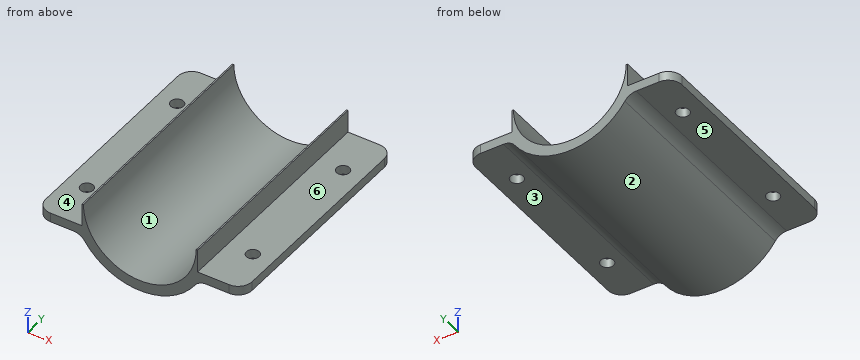
from build123d import *

# Parameters (mm, degrees)
BOSS_EXTRUDE1_DEPTH = 50
SKETCH2_R           = 1.4
CUT_EXTRUDE3_DEPTH  = 2
FILLET2_R           = 3


with BuildPart() as part:
    # Sketch1 → Boss-Extrude1 (new body)
    with BuildSketch(Plane(origin=(0, 0, 0), x_dir=(1, 0, 0), z_dir=(0, 1, 0))):
        with BuildLine():
            Line((-12.6, 0), (-12.6, 5))
            Line((-12.6, 5), (-22.5, 5))
            Line((-22.5, 5), (-22.5, 7))
            Line((-22.5, 7), (-22.1, 7))
            Line((-22.1, 7), (-14.483093592, 7))
            ThreePointArc((-14.483093592, 7), (-13.089113026, 7.343532763), (-12.014384457, 8.295454545))
            ThreePointArc((-12.014384457, 8.295454545), (0, 14.6), (12.014384457, 8.295454545))
            ThreePointArc((12.014384457, 8.295454545), (13.089113026, 7.343532763), (14.483093592, 7))
            Line((14.483093592, 7), (22.1, 7))
            Line((22.1, 7), (22.5, 7))
            Line((22.5, 7), (22.5, 5))
            Line((22.5, 5), (12.6, 5))
            Line((12.6, 5), (12.6, 0))
            Line((12.6, 0), (12.3, 0))
            ThreePointArc((12.3, 0), (0, 12.3), (-12.3, 0))
            Line((-12.3, 0), (-12.6, 0))
        make_face()
    extrude(amount=BOSS_EXTRUDE1_DEPTH)

    # Sketch2 → Cut-Extrude3 (cut)
    with BuildSketch(Plane(origin=(0, 0, -7), x_dir=(-1, 0, 0), z_dir=(0, 0, -1))):
        with Locations((-18.1, 10)):
            Circle(SKETCH2_R)
        with Locations(Location((-18.1, 40, 0), (0, 0, 180))):
            Circle(SKETCH2_R)
        with Locations((18.1, 40)):
            Circle(SKETCH2_R)
        with Locations(Location((18.1, 10, 0), (0, 0, 180))):
            Circle(SKETCH2_R)
    extrude(amount=-CUT_EXTRUDE3_DEPTH, mode=Mode.SUBTRACT)

    # Fillet2
    fillet2_edges = [part.edges().sort_by_distance(p)[0] for p in [
        (-22.5, 0, -6),
        (22.5, 0, -6),
        (22.5, 50, -6),
        (-22.5, 50, -6),
    ]]
    fillet(fillet2_edges, radius=FILLET2_R)


solid = part.part
Could you check a few things on this model? Use its own coordinates, in mm. Face numbers are marked on the shaded views. A direction names the side the tool comes from. Coordinates: 2 decimals unless noted, no trailing zeros. Loops run counter-clockwise (first coordinate to the right, second up) from the corner with the lowest first, then second, coordinate; pieces in that order, holes last. Notation, with made-up numbers: (-19.5, 74.25) -> (22.5, 74.25) arc R9 ccw to (22.5, 90.25) -> close; hole circle Ø6 at (57.5, -31.5). An arc over 180 degrees is marked (long way). Answer in a Markdown table with one row per item.
(1) If I drill on probe 1 along Y at (x, z) = (-18.1, -5.85); probe 2 along X at (y, z) = (41, -9.5); probe 3 along Z at (x, y) = (21, 41.5), over which ranges is the centre line in solid material (lowest first)?
Results found:
| item | result |
|---|---|
| probe 1 | y = 0 to 8.6, 11.4 to 38.6, 41.4 to 50 |
| probe 2 | x = -11.09 to -7.81, 7.81 to 11.09 |
| probe 3 | z = -7 to -5 |
(2) For the marked faces 4, 5 and 6, which set-ups out of +Z, -Z, +X, -X, +Y, -Y let a thin tool reach every point of the face, with its end or its side?
Results found:
| item | result |
|---|---|
| face 4 | +Z, -X, +Y, -Y |
| face 5 | -Z, -X, +Y, -Y |
| face 6 | +Z, +X, +Y, -Y |
(3) Imagine slicing it at C-C (y = 40). List the corners of the cut face in (x, z) for me, plus the area to 3 significant figures.
Results found:
| item | result |
|---|---|
| outline | (-22.5, -7) -> (-19.5, -7) -> (-19.5, -5) -> (-22.5, -5) -> close; (-16.7, -7) -> (-14.48, -7) arc R3 cw to (-12.01, -8.3) arc R14.6 ccw to (12.01, -8.3) arc R3 cw to (14.48, -7) -> (16.7, -7) -> (16.7, -5) -> (12.6, -5) -> (12.6, 0) -> (12.3, 0) arc R12.3 cw to (-12.3, 0) -> (-12.6, 0) -> (-12.6, -5) -> (-16.7, -5) -> close; (19.5, -7) -> (22.5, -7) -> (22.5, -5) -> (19.5, -5) -> close |
| area | 107 mm^2 |
(4) Imagine slicing it at A-A (x = -18.1). List the corners of the cut face in (y, z) for me.
Results found:
| item | result |
|---|---|
| outline | (0, -7) -> (8.6, -7) -> (8.6, -5) -> (0, -5) -> close; (11.4, -7) -> (38.6, -7) -> (38.6, -5) -> (11.4, -5) -> close; (41.4, -7) -> (50, -7) -> (50, -5) -> (41.4, -5) -> close |
(5) Imagine slicing it at D-D (y = 25). List the corners of the cut face in (x, z) for me, plus the area to 3 significant figures.
Results found:
| item | result |
|---|---|
| outline | (-22.5, -7) -> (-14.48, -7) arc R3 cw to (-12.01, -8.3) arc R14.6 ccw to (12.01, -8.3) arc R3 cw to (14.48, -7) -> (22.5, -7) -> (22.5, -5) -> (12.6, -5) -> (12.6, 0) -> (12.3, 0) arc R12.3 cw to (-12.3, 0) -> (-12.6, 0) -> (-12.6, -5) -> (-22.5, -5) -> close |
| area | 118 mm^2 |
(6) Will these pins go through, and if not, where does the flat tip stop? pin 1 Ø11 at (x, y) = (18, 15) entering from +Z; pin 2 Ø3 at (x, y) = (18.1, 10) entering from -Z; pin 3 Ø10 at (x, y) = (0.5, 26) entering from +Z; pin 4 Ø3.5 at (x, y) = (-18.1, 10) entering from +Z.
Results found:
| item | result |
|---|---|
| pin 1 | stops at z = 0 |
| pin 2 | stops at z = -7 |
| pin 3 | stops at z = -11 |
| pin 4 | stops at z = -5 |
(7) Imagine slicing it at B-B (z = -5.75). List the corners of the cut face in (x, y) for me, plus the area to 3 significant figures.
Results found:
| item | result |
|---|---|
| outline | (-22.5, 3) arc R3 ccw to (-19.5, 0) -> (-10.87, 0) -> (-10.87, 50) -> (-19.5, 50) arc R3 ccw to (-22.5, 47) -> close; (10.87, 0) -> (19.5, 0) arc R3 ccw to (22.5, 3) -> (22.5, 47) arc R3 ccw to (19.5, 50) -> (10.87, 50) -> close; hole circle Ø2.8 at (-18.1, 10); hole circle Ø2.8 at (-18.1, 40); hole circle Ø2.8 at (18.1, 10); hole circle Ø2.8 at (18.1, 40) |
| area | 1,130 mm^2 |
(8) Thinking about a two-plate mould opening in X: for the marked faces 1, 2 and 3, which applies, released by +X, released by -X, zero draft, split by the parting line, or undercut?
Results found:
| item | result |
|---|---|
| face 1 | undercut |
| face 2 | split by the parting line |
| face 3 | zero draft |
